Autodesk Inventor part; units mm, degrees
ref_plane "YZ Plane" through (0, 0, 0) normal (1, 0, 0) x (0, 1, 0)
ref_plane "XZ Plane" through (0, 0, 0) normal (0, 1, 0) x (-1, 0, 0)
ref_plane "XY Plane" through (0, 0, 0) normal (0, 0, 1) x (1, 0, 0)
sketch "Sketch1" plane through (0, 0, 0) normal (0, 1, 0) x (-1, 0, 0)
  line L0 (0, 0) -> (0, 4.6)
  line L1 (0, 4.6) -> (14, 4.6) construction
  line L2 (14, 4.6) -> (16.5, 4.6)
  line L3 (16.5, 4.6) -> (16.5, 1)
  line L4 (16.5, 1) -> (23, 1)
  line L5 (23, 1) -> (23, 0)
  line L6 (23, 0) -> (15.5, 0)
  line L7 (15.5, 0) -> (0, 0) construction
  line L8 (14, 4.6) -> (14, 3.6)
  line L9 (14, 3.6) -> (15.5, 3.6)
  line L10 (15.5, 3.6) -> (15.5, 0)
  dimension "d0" = 46
  dimension "d2" = 31
  dimension "d3" = 28
  dimension "d4" = 3.6
  dimension "d5" = 1
  dimension "d6" = 1
  dimension "d7" = 1
revolve "Revolution1" add sketch "Sketch1" angle 360 about axis through (0, 0, 0) along (0, 0, 1)
sketch "Sketch2" plane through (0, 0, 1) normal (0, 0, 1) x (1, 0, 0)
  circle A0 centre (0, 0) radius 20.5 construction
  line L0 (-14.4957, 14.4957) -> (0, 0) construction
  line L1 (0, 0) -> (-12.5096, 0) construction
  dimension "d9" = 41
  dimension "d20" = 45
hole "Hole1" at (-14.4957, 14.4957, 1) direction (0, 0, -1) diameter 3.2 end through all
pattern_circular "Circular Pattern1" count 4 over 360 about axis through (0, 0, 0.5) along (0, 0, 1) of "Hole1"
sketch "Sketch3" plane through (0, 0, 0) normal (0, 0, 1) x (1, 0, 0)
  line L0 (-28.4447, -15.8605) -> (-21, -15.8605)
  line L1 (-21, -15.8605) -> (-21, 15.8605)
  line L2 (-21, 15.8605) -> (-28.4447, 15.8605)
  line L3 (-28.4447, 15.8605) -> (-28.4447, -15.8605)
  point P0 (0, 0)
  point P1 (-28.4447, 0)
  dimension "d21" = 21
extrude "Extrusion1" cut sketch "Sketch3" along normal through all
fillet "Fillet1" radius 10 2 edges at (-21, -9.3808, 0.5) (-21, 9.3808, 0.5)
mirror "Mirror1" about plane through (0, 0, 0) normal (1, 0, 0) of "Extrusion1", "Fillet1"
equation "\"d5\" = wall_thickness"
equation "\"d6\" = wall_thickness"
equation "\"d7\" = wall_thickness"
equation "\"wall_thickness\" = 1"
properties part number "quartz-disk-window-holder" material "Stainless Steel"
Can you work these out from the model? Positions are in its coordinate system, mm. A direction names the side the tool comes from. Round coordinates to 2 decimals unless told otherwise and drop trailing zeros. Order: outer loops, then holes, each group sorted by start corner. A loop starts at its lowest first (then second) coordinate and runs counter-clockwise, first axis right, second up. Notation, with made-up numbers: (9.5, 88) - (14.5, 88) arc R23 ccw to (14.5, 126) - close; hole circle Ø3 at (74, 50.5). An arc over 180 degrees is marked (long way). Answer in a Markdown table with one row per item.
(1) If we mould it in two halves opening along X, with no side actions, what happens to faces 4 (the face through (20.62, -9.66, 0.49)), 5 (the face through (0.3, -23, 0.5)), 6 (the face through (-12.932, -5.362, 4.093))? For each: released by +X, released by -X, zero draft, split by the parting line, or undercut.
From the geometry:
| item | result |
|---|---|
| face 4 | released by +X |
| face 5 | split by the parting line |
| face 6 | undercut |
(2) Suppose I cut it at D-D, the plane y = 20. Please give me the cut outline in (x, z).
From the geometry:
| item | result |
|---|---|
| outline | (-11.36, 0) - (11.36, 0) - (11.36, 1) - (-11.36, 1) - close |
(3) Suppose I cut it at C-C, the plane z = 1.6. Please give me the cut outline in (x, y), plus the area to 3 significant figures.
From the geometry:
| item | result |
|---|---|
| outline | circle Ø33 at (0, 0); hole circle Ø31 at (0, 0) |
| area | 101 mm2 |
(4) Suppose I cut it at A-A, the plane y = 0. Please give me the cut outline in (x, z).
From the geometry:
| item | result |
|---|---|
| outline | (-21, 0) - (-15.5, 0) - (-15.5, 3.6) - (-14, 3.6) - (-14, 4.6) - (-16.5, 4.6) - (-16.5, 1) - (-21, 1) - close; (14, 3.6) - (15.5, 3.6) - (15.5, 0) - (21, 0) - (21, 1) - (16.5, 1) - (16.5, 4.6) - (14, 4.6) - close |
(5) For P1, Ø4, axis at x = 14.5, y = 14.5, coming from the +Z side; P2, Ø9.5, axis at x = -4, y = 7, coming from the -Z side, each with a flat end and sliding along its axis, tell me the tip position at first contact or that it passes through.
From the geometry:
| item | result |
|---|---|
| P1 | stops at z = 1 |
| P2 | passes through |
(6) Please list where these lines run through material, in increasing order: L1, parallel to X at y = 0, z = 4.1; L2, parallel to Y at x = -4.5, z = 2.9. Write a range as from..to.
From the geometry:
| item | result |
|---|---|
| L1 | x = -16.5..-14, 14..16.5 |
| L2 | y = -15.87..-14.83, 14.83..15.87 |
(7) Which directions (+Z, -Z, +X, -X, +Y, -Y) give clear straight access to the entire face, cutting with the end or side of a thin tool? Please do faces 1 (the face through (-13.076, 13.757, 0.493)), 2 (the face through (2.018, 15.368, 1.775)), 3 (the face through (16, -5, 1)).
From the geometry:
| item | result |
|---|---|
| face 1 | +Z, -Z |
| face 2 | -Z |
| face 3 | +Z |
(8) Suppose I cut it at B-B, the plane x = 0. Please give me the cut outline in (y, z).
From the geometry:
| item | result |
|---|---|
| outline | (-23, 0) - (-15.5, 0) - (-15.5, 3.6) - (-14, 3.6) - (-14, 4.6) - (-16.5, 4.6) - (-16.5, 1) - (-23, 1) - close; (14, 3.6) - (15.5, 3.6) - (15.5, 0) - (23, 0) - (23, 1) - (16.5, 1) - (16.5, 4.6) - (14, 4.6) - close |
